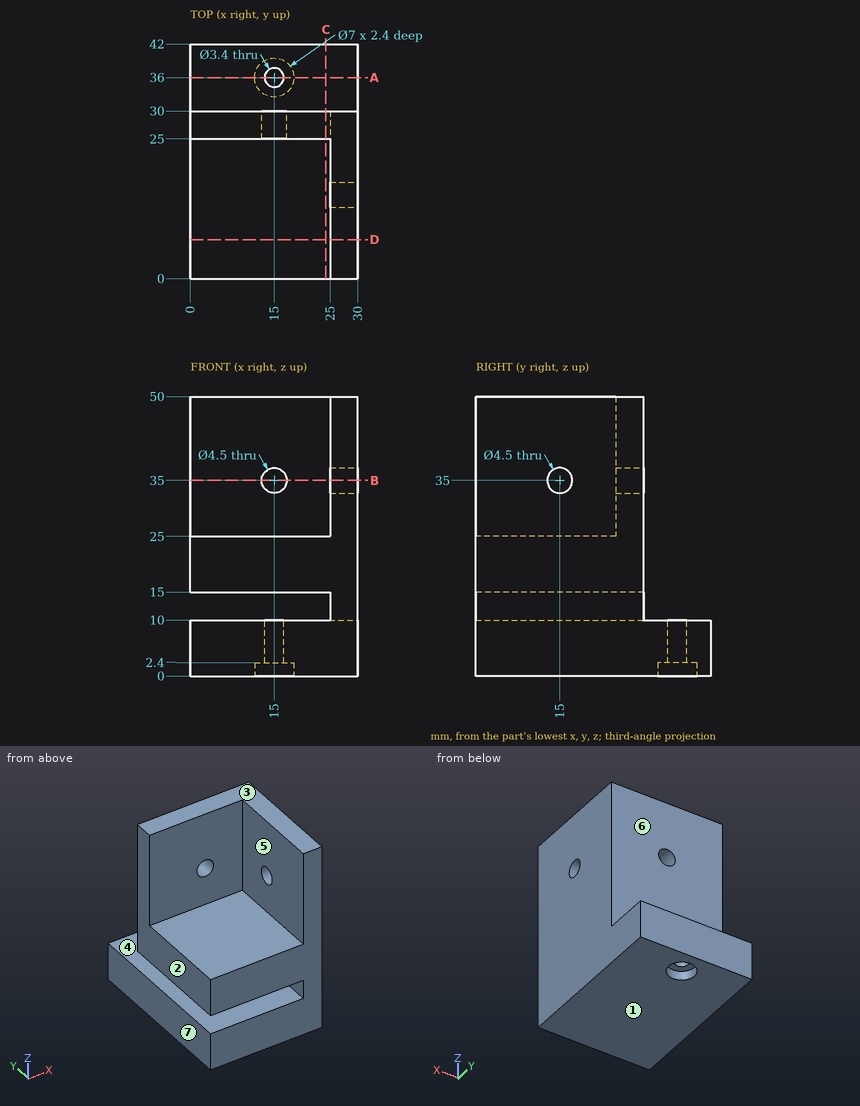
Job drawing, mm, ordinate dimensions from the low corner. One solid piece. A direction names the side the tool comes from. Give positions to 0.01 mm unless a question says otherwise; leave off trailing zeros. Order: outer loops, then holes, each group sorted by start corner. A loop starts at its lowest first (then second) coordinate and runs counter-clockwise, first axis right, second up. Notation, with made-up numbers: M -40,36 L 15,36 A33 ccw 15,68 Z; hole C 82.25,-23.5 d5. An arc over 180 degrees is marked long. Put each result on its own line as item: value. Start each with the question number.
(1) Pin check, flat tips, straight feed: pin 1 Ø12.5 at (x, z) = (10, 33.5) entering from -Y; pin 2 Ø8 at (x, z) = (19, 41) entering from +Y; pin 3 Ø4.5 at (x, y) = (15, 36) entering from +Z. Stop position of each tip, or through.
(2) Band-saw the part on C-C on x = 24.25. Give the cut face in (y, z), then the cut area to 3 significant figures.
(3) Band-saw the part on D-D on y = 7. Give the cut face in (x, z).
(4) Drill centre lines: L1, parallel to Y at x = 15, z = 4.5; L2, parallel to Z at x = 2, y = 11.5; L3, parallel to Y at x = 15, z = 1.6. Where is each one in solid material? Low to high. Write a range as [from, to].
(5) Tool access for the marked faces 5, 6 and 7: list every direction of +Z, -Z, +X, -X, +Y, -Y with a clear straight run to the whole face (end or side of a thin tool).
(6) Pull direction Z, two halves, no side cores. Call the marked faces 1, 2, 3 and 4: released by +Z, released by -Z, zero draft, split by the parting line, or undercut.
(7) Band-saw the part on A-A on y = 36. Give the cut face in (x, z), then the cut area to 3 significant figures.
(8) Band-saw the part on B-B on z = 35. Give the cut face in (x, y), then the cut area to 3 significant figures.
Results below:
1. pin 1: stops at y = 25
1. pin 2: stops at y = 30
1. pin 3: stops at z = 10
2. outline: M 0,0 L 42,0 L 42,10 L 0,10 Z; M 0,15 L 30,15 L 30,50 L 25,50 L 25,25 L 0,25 Z
2. area: 845 mm2
3. outline: M 0,0 L 30,0 L 30,50 L 25,50 L 25,25 L 0,25 L 0,15 L 25,15 L 25,10 L 0,10 Z
4. L1: y = [0, 34.3], [37.7, 42]
4. L2: z = [0, 10], [15, 25]
4. L3: y = [0, 32.5], [39.5, 42]
5. face 5: +Z, -X, -Y
5. face 6: +Z, +X, -X, +Y
5. face 7: +Z, -Z, -X, +Y, -Y
6. face 1: released by -Z
6. face 2: zero draft
6. face 3: released by +Z
6. face 4: undercut
7. outline: M 0,0 L 11.5,0 L 11.5,2.4 L 13.3,2.4 L 13.3,10 L 0,10 Z; M 16.7,2.4 L 18.5,2.4 L 18.5,0 L 30,0 L 30,10 L 16.7,10 Z
7. area: 257 mm2
8. outline: M 0,25 L 12.75,25 L 12.75,30 L 0,30 Z; M 17.25,25 L 25,25 L 25,17.25 L 30,17.25 L 30,30 L 17.25,30 Z; M 25,0 L 30,0 L 30,12.75 L 25,12.75 Z
8. area: 230 mm2
